Model file for the job. Use its own axes, mm. Face numbers are marked on the shaded views. A direction names the side the tool comes from. Round coordinates to 2 decimals unless told otherwise and drop trailing zeros. Loops run counter-clockwise (first coordinate to the right, second up) from the corner with the lowest first, then second, coordinate; pieces in that order, holes last. Notation, with made-up numbers: (-18, 41.25) - (25, 41.25) arc R24 cw to (25, 71.25) - close; hole circle Ø7 at (38.5, 28). An arc over 180 degrees is marked (long way). Use one line per item in the form item = value.
from build123d import *

# Parameters (mm, degrees)
SKETCH3_R          = 0.75
CUT_EXTRUDE1_DEPTH = 75
SKETCH4_R          = 1
CUT_EXTRUDE2_DEPTH = 5


with BuildPart() as part:
    # Sketch1 → Revolve1 (revolve)
    with BuildSketch(Plane(origin=(0, 0, 0), x_dir=(0, 0, -1), z_dir=(1, 0, 0))):
        with BuildLine():
            Line((0, 80), (10, 80))
            Line((10, 80), (10, 75))
            Line((10, 75), (7.5, 75))
            Line((7.5, 75), (7.5, 30))
            Line((7.5, 30), (2.2, 30))
            Line((2.2, 30), (2.2, 6.707802986))
            add(Edge.make_bspline(
                [(5.5, 3.5), (5.5, 5.791287847), (2.2, 6.707802986)],
                knots=[3.141592654, 3.141592654, 3.141592654, 4.300872134, 4.300872134, 4.300872134], degree=2, weights=[1, 0.836660027, 1]))
            Line((5.5, 3.5), (5.5, 0))
            Line((5.5, 0), (4.5, 0))
            Line((4.5, 0), (4.5, 1))
            Line((4.5, 1), (4.5, 3.5))
            add(Edge.make_bspline(
                [(4.5, 3.5), (4.5, 3.697156866), (4.420178962, 4.058188281), (3.970108568, 4.705926092), (3.267562051, 5.215959335), (2.550576032, 5.549361773), (2.137087255, 5.687424721), (1.93239721, 5.744273668)],
                knots=[3.141592654, 3.141592654, 3.141592654, 3.141592654, 3.431412524, 3.721232394, 4.011052264, 4.155962199, 4.300872134, 4.300872134, 4.300872134, 4.300872134], degree=3))
            Line((1.93239721, 5.744273668), (0, 5.744273668))
            Line((0, 5.744273668), (0, 80))
        make_face()
    revolve(axis=Axis((0, 5.744273668, 0), (0, 1, 0)))

    # Sketch3 → Cut-Extrude1 (cut)
    with BuildSketch(Plane.XZ.offset(-5.744273668)):
        with Locations(Location((0, 0, 0), (0, 0, 270))):
            Circle(SKETCH3_R)
    extrude(amount=-CUT_EXTRUDE1_DEPTH, mode=Mode.SUBTRACT)

    # Sketch4 → Cut-Extrude2 (cut)
    with BuildSketch(Plane(origin=(0, 80, 0), x_dir=(1, 0, 0), z_dir=(0, 1, 0))):
        with Locations(Location((-2.985595387, 7.528271622, 0), (0, 0, 270))):
            Circle(SKETCH4_R)
        with Locations(Location((3.212157171, 7.434426659, 0), (0, 0, 270))):
            Circle(SKETCH4_R)
        with Locations(Location((7.528271622, 2.985595387, 0), (0, 0, 270))):
            Circle(SKETCH4_R)
        with Locations(Location((7.434426659, -3.212157171, 0), (0, 0, 270))):
            Circle(SKETCH4_R)
        with Locations(Location((2.985595387, -7.528271622, 0), (0, 0, 270))):
            Circle(SKETCH4_R)
        with Locations(Location((-3.212157171, -7.434426659, 0), (0, 0, 270))):
            Circle(SKETCH4_R)
        with Locations(Location((-7.528271622, -2.985595387, 0), (0, 0, 270))):
            Circle(SKETCH4_R)
        with Locations(Location((-7.434426659, 3.212157171, 0), (0, 0, 270))):
            Circle(SKETCH4_R)
    extrude(amount=-CUT_EXTRUDE2_DEPTH, mode=Mode.SUBTRACT)


solid = part.part
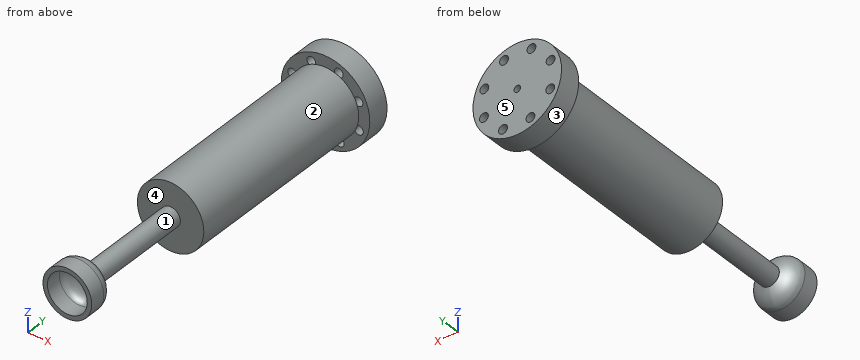
1. Cut at A-A, the plane y = 25.5. Give the cut face in (x, z).
Geometry check:
outline = circle Ø4.4 at (0, 0); hole circle Ø1.5 at (0, 0)
2. Cut at B-B, the plane y = 59. Give the cut face in (x, z).
Geometry check:
outline = circle Ø15 at (0, 0); hole circle Ø1.5 at (0, 0)
3. Tool access for the marked faces 1 and 2: list every direction of +Z, -Z, +X, -X, +Y, -Y with a clear straight run to the whole face (end or side of a thin tool).
Geometry check:
face_1 = none
face_2 = -Y
4. Flat gauge pins, fed straight in: pin 1 (3 mm diameter, centred on x = -7.5, y = 63.5, fed in from +Z); pin 2 (2.5 mm diameter, centred on x = 0, z = 0, fed in from -Y); pin 3 (2.5 mm diameter, centred on x = -2.99, z = -7.53, fed in from -Y); pin 4 (2.5 mm diameter, centred on x = -7.53, z = 2.99, fed in from +Y). Where does each tip first touch, or does it go through?
Geometry check:
pin_1 = 4.5
pin_2 = 5.74
pin_3 = 30
pin_4 = 80
5. Pull direction Y, two halves, no side cores. Call the marked faces 3, 4 and 5: +Y half, -Y half, draft (parallel to the pull), parting line (faces both ways), or undercut.
Geometry check:
face_3 = draft
face_4 = undercut
face_5 = +Y half
6. Wall check: probe 1 along Z at (x, y) = (2, 69); probe 2 along Z at (x, y) = (0.5, 66.5); probe 3 along Y at (x, z) = (0.25, -4.75). Give the ranges that are in metal, low to high.
Geometry check:
probe_1 = -7.23 to 7.23
probe_2 = -7.48 to -0.56, 0.56 to 7.48
probe_3 = 0 to 5.26, 30 to 80
